Input: dimensioned drawing with shaded views. Units: mm. Origin: part minimum x, y, z. A direction names the side the tool comes from. Coordinates: 2 decimals unless noted, no trailing zeros. Write each loop counter-clockwise with the first axis right and the second up, starting at its lowest first coordinate (ties: lowest second). Pieces come first, ordered by that corner, then holes. Notation, with made-up numbers: M 51.25,34 L 82.25,34 A18 cw 82.25,43 Z; hole C -15.75,-9 d8. An arc over 180 degrees is marked long. Write each question's results on one line, items separated by ' | '. Start each with the question number.
1. Pull-direction query (Z, two-part tool) for the marked faces 1, 2, 3 and 4; classes: +Z half, -Z half, draft (parallel to the pull), parting line (faces both ways), or undercut.
2. Section query C-C, the plane z = 22. Output: boundary loops of the cut face in (x, y), and give its area (3 significant figures).
3. Set-up query: the marked faces 5, 6, 7 and 8. Return all of +Z, -Z, +X, -X, +Y, -Y with unobstructed straight access to the full face (end or side cutting, diameter ignored); none if empty.
4. Section query B-B, the plane z = 30. Count the separate pieces of the cut face and the enclosed holes in it, and give its area (3 significant figures).
5. Section query D-D, the plane x = 56.5. Output: boundary loops of the cut face in (y, z), and give its area (3 significant figures).
6. Section query A-A, the plane x = 30. Output: boundary loops of the cut face in (y, z), and give its area (3 significant figures).
7. Ray query, probe 1 along X at (y, z) = (1.8, 15); probe 2 along Z at (x, y) = (29.5, 10); probe 3 along Z at (x, y) = (11.9, 20). Return the intervals inside material, ascending.
8. First-contact query: pin 1 (5 mm diameter, centred on x = 56.5, z = 45, fed in from +Y); pin 2 (3 mm diameter, centred on x = 41.5, y = 15, fed in from -Z); pin 3 (12 mm diameter, centred on y = 17.5, z = 31.5, fed in from -X); pin 4 (3.5 mm diameter, centred on y = 20, z = 30, fed in from +X). Flat tips, straight axial feed; report the tip coordinate or a pass-through.
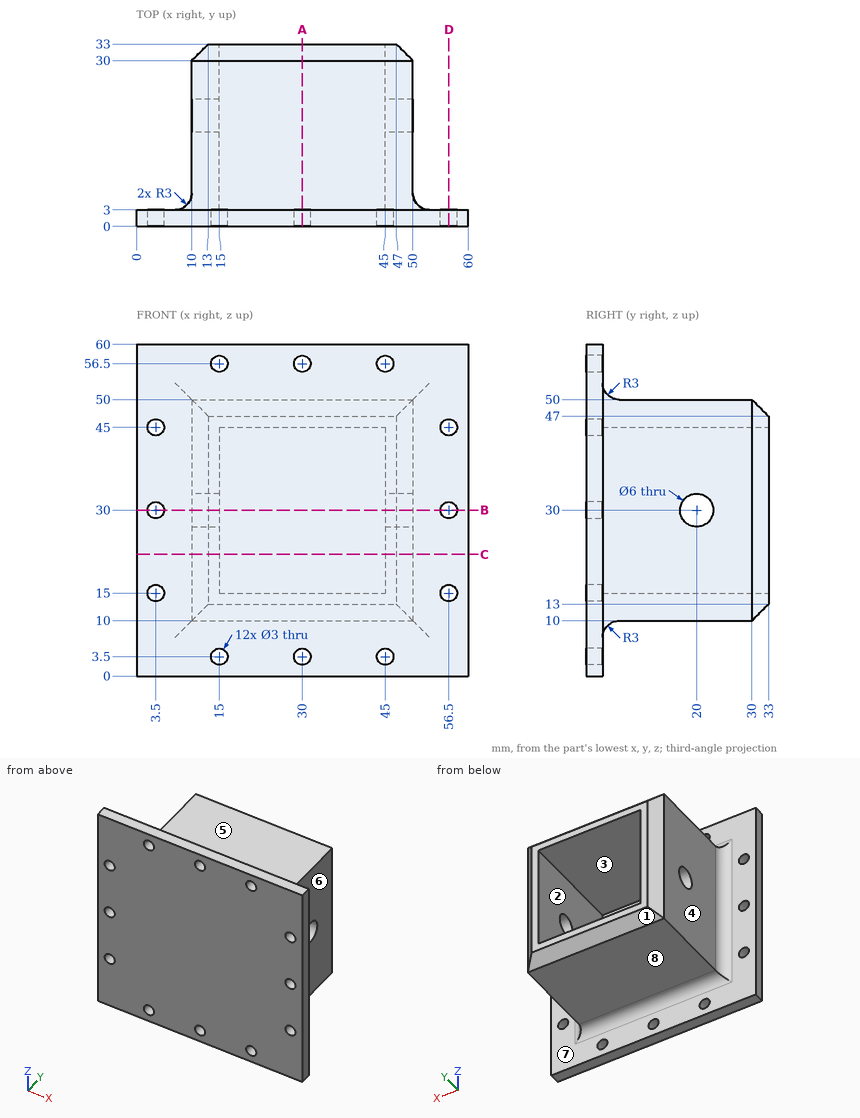
Answer:
1) face 1: -Z half | face 2: undercut | face 3: undercut | face 4: draft
2) outline: M 0,0 L 60,0 L 60,3 L 53,3 A3 cw 50,6 L 50,30 L 47,33 L 45,33 L 45,3 L 15,3 L 15,33 L 13,33 L 10,30 L 10,6 A3 cw 7,3 L 0,3 Z | area: 475 mm^2
3) face 5: +Z, +X, -X, +Y | face 6: +Z, -Z, +X, +Y | face 7: +Y | face 8: -Z, +X, -X, +Y
4) separate pieces: 5 | enclosed holes: 0 | area: 397 mm^2
5) outline: M 0,0 L 3,0 L 3,13.5 L 0,13.5 Z; M 0,16.5 L 3,16.5 L 3,28.5 L 0,28.5 Z; M 0,31.5 L 3,31.5 L 3,43.5 L 0,43.5 Z; M 0,46.5 L 3,46.5 L 3,60 L 0,60 Z | area: 153 mm^2
6) outline: M 0,0 L 3,0 L 3,2 L 0,2 Z; M 0,5 L 3,5 L 3,7 A3 cw 6,10 L 30,10 L 33,13 L 33,15 L 3,15 L 3,45 L 33,45 L 33,47 L 30,50 L 6,50 A3 cw 3,53 L 3,55 L 0,55 Z; M 0,58 L 3,58 L 3,60 L 0,60 Z | area: 457 mm^2
7) probe 1: 0 to 2, 5 to 55, 58 to 60 | probe 2: 10 to 15, 45 to 50 | probe 3: 10 to 27, 33 to 50
8) pin 1: y = 3 | pin 2: z = 10 | pin 3: x = 10 | pin 4: through
